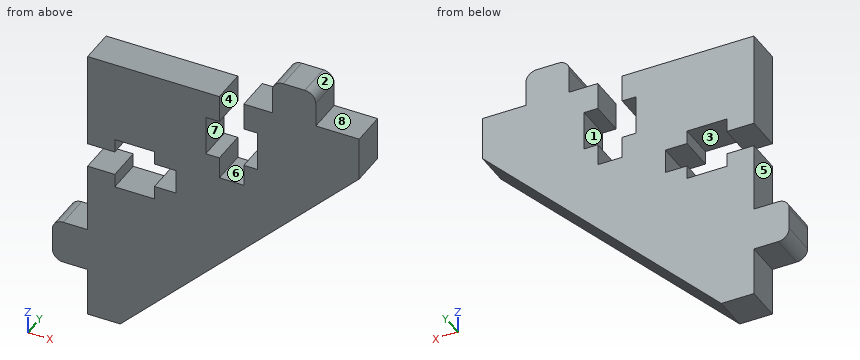
Autodesk Inventor part; units mm, degrees
ref_plane "YZ Plane" through (0, 0, 0) normal (1, 0, 0) x (0, 1, 0)
ref_plane "XZ Plane" through (0, 0, 0) normal (0, 1, 0) x (-1, 0, 0)
ref_plane "XY Plane" through (0, 0, 0) normal (0, 0, 1) x (1, 0, 0)
sketch "Sketch1" plane through (0, 0, 0) normal (0, 1, 0) x (-1, 0, 0)
  line L0 (0, -51.7) -> (0, 0)
  line L1 (0, 0) -> (-50, 0)
  line L2 (-50, 0) -> (-50, -8)
  line L3 (-50, -8) -> (-6, -51.7)
  line L4 (-6, -51.7) -> (0, -51.7)
  dimension "d0" = 51.7
  dimension "d1" = 50
  dimension "d2" = 8
  dimension "d3" = 6
extrude "Extrusion1" add sketch "Sketch1" along normal blind 6.5
sketch "Sketch2" plane through (0, 6.5, 0) normal (0, 1, 0) x (1, 0, 0)
  line L0 (0, 0) -> (50, 0)
  line L1 (50, 0) -> (50, 8)
  line L2 (34, 0) -> (42, 0)
  line L3 (42, 0) -> (42, -4.5)
  line L4 (40, -6.5) -> (36, -6.5)
  line L5 (34, -4.5) -> (34, 0)
  arc A0 (34, -4.5) -> (36, -6.5) centre (36, -4.5) ccw
  arc A1 (40, -6.5) -> (42, -4.5) centre (40, -4.5) ccw
  dimension "d6" = 2
  dimension "d7" = 8
  dimension "d8" = 6.5
  dimension "d9" = 8
extrude "Extrusion2" add sketch "Sketch2" against normal blind 6.5
sketch "Sketch3" plane through (0, 6.5, 0) normal (0, 1, 0) x (1, 0, 0)
  line L0 (0, 0) -> (34, 0)
  line L1 (34, 0) -> (34, -4.5)
  line L2 (24.25, 16.3) -> (28.75, 16.3)
  line L3 (28.75, 0) -> (24.25, 0)
  line L4 (31.25, 12.3) -> (31.25, 5)
  line L5 (21.75, 5) -> (21.75, 12.3)
  line L6 (21.75, 12.3) -> (24.25, 12.3)
  line L7 (28.75, 12.3) -> (31.25, 12.3)
  line L8 (24.25, 0) -> (24.25, 5)
  line L9 (24.25, 12.3) -> (24.25, 16.3)
  line L10 (31.25, 5) -> (28.75, 5)
  line L11 (24.25, 5) -> (21.75, 5)
  line L12 (28.75, 16.3) -> (28.75, 12.3)
  line L13 (28.75, 5) -> (28.75, 0)
  point P0 (26.5, 16.3)
  dimension "d12" = 4.5
  dimension "d13" = 5
  dimension "d14" = 7.3
  dimension "d15" = 4
  dimension "d16" = 2.5
  dimension "d17" = 7.5
extrude "Extrusion3" cut sketch "Sketch3" against normal through all
sketch "Sketch4" plane through (0, 6.5, 0) normal (0, 1, 0) x (1, 0, 0)
  line L0 (0, 51.7) -> (0, 0)
  line L1 (0, 0) -> (24.25, 0)
  line L2 (16.3, 22) -> (16.3, 17.5)
  line L3 (0, 17.5) -> (0, 22)
  line L4 (5, 24.5) -> (12.3, 24.5)
  line L5 (12.3, 15) -> (5, 15)
  line L6 (0, 22) -> (5, 22)
  line L7 (12.3, 22) -> (16.3, 22)
  line L8 (16.3, 17.5) -> (12.3, 17.5)
  line L9 (5, 17.5) -> (0, 17.5)
  line L10 (5, 15) -> (5, 17.5)
  line L11 (5, 22) -> (5, 24.5)
  line L12 (12.3, 24.5) -> (12.3, 22)
  line L13 (12.3, 17.5) -> (12.3, 15)
  point P0 (16.3, 19.75)
  dimension "d20" = 4.5
  dimension "d21" = 5
  dimension "d22" = 4
  dimension "d23" = 7.3
  dimension "d24" = 19.75
  dimension "d25" = 2.5
extrude "Extrusion4" cut sketch "Sketch4" against normal through all
sketch "Sketch5" plane through (0, 6.5, 0) normal (0, 1, 0) x (1, 0, 0)
  line L0 (16.3, 22) -> (16.3, 17.5)
  line L1 (0, 51.7) -> (0, 22)
  line L2 (0, 42.75) -> (-4.5, 42.75)
  line L3 (-6.5, 40.75) -> (-6.5, 36.75)
  line L4 (-4.5, 34.75) -> (0, 34.75)
  line L5 (0, 34.75) -> (0, 42.75)
  arc A0 (-4.5, 42.75) -> (-6.5, 40.75) centre (-4.5, 40.75) ccw
  arc A1 (-6.5, 36.75) -> (-4.5, 34.75) centre (-4.5, 36.75) ccw
  point P0 (16.3, 19.75)
  dimension "d28" = 2
  dimension "d29" = 8
  dimension "d30" = 6.5
  dimension "d31" = 15
extrude "Extrusion5" add sketch "Sketch5" against normal blind 6.5
properties part number "x_carryage_brace_top"
The listing builds one solid part. Answer for the finished solid, in the listing's coordinates (mm). Face numbers are marked on the shaded views. A direction names the side the tool comes from. Give positions to 0.01 mm unless a question says otherwise; leave off trailing zeros. Loops run counter-clockwise (first coordinate to the right, second up) from the corner with the lowest first, then second, coordinate; pieces in that order, holes last. Notation, with made-up numbers: (54, 61) - (107, 61) arc R25 ccw to (107, 98) - close; hole circle Ø1 at (-2, 87.5). An arc over 180 degrees is marked (long way). Answer as CSV lines item,"result". Start each with the question number.
Item 1: A cutting plane is placed at B-B on x = 9. Determine the outline of the cut face in (y, z).
Item 2: Find the intervals of material crossed by line 1 (X direction, y = 5.25, z = -4); line 2 (Z direction, x = 29.5, y = 4); line 3 (Z direction, x = 23.5, y = 4.25), in increasing order. Write a range as from..to.
Item 3: A cutting plane is placed at D-D on z = -45.5. Determine the outline of the cut face in (x, y).
Item 4: The mould has two halves that part along Z. Classify the marked faces 1, 2, 3 and 4: +Z half, -Z half, draft (parallel to the pull), parting line (faces both ways), or undercut.
Item 5: A cutting plane is placed at C-C on x = -1. Determine the outline of the cut face in (y, z), then the cut area to 3 significant figures.
Item 6: For the marked faces 5, 6, 7 and 8, determine the directions among +Z, -Z, +X, -X, +Y, -Y from which every point of the face is accessible in a straight line to the end or side of a thin tool.
Item 7: Each of these flat-tipped pins is pushed along its axis until it touches: pin 1 (2 mm diameter, centred on y = 4.5, z = -45.5, fed in from -X); pin 2 (2 mm diameter, centred on y = 2, z = -19, fed in from -X); pin 3 (2 mm diameter, centred on x = 47.5, y = 4.5, fed in from +Z). Where does it stop, or does it pass through?
Item 8: A cutting plane is placed at A-A on z = -3. Determine the outline of the cut face in (x, y).
Found:
1,outline,"(0, -48.72) - (6.5, -48.72) - (6.5, -24.5) - (0, -24.5) - close; (0, -15) - (6.5, -15) - (6.5, 0) - (0, 0) - close"
2,line 1,"x = 0..24.25, 28.75..50"
2,line 2,"z = -28.36..-12.3, -5..0"
2,line 3,"z = -34.32..-12.3, -5..0"
3,outline,"(0, 0) - (12.24, 0) - (12.24, 6.5) - (0, 6.5) - close"
4,face 1,"undercut"
4,face 2,"+Z half"
4,face 3,"undercut"
4,face 4,"draft"
5,outline,"(0, -42.75) - (6.5, -42.75) - (6.5, -34.75) - (0, -34.75) - close"
5,area,"52.0 mm^2"
6,face 5,"+Z, -X, +Y, -Y"
6,face 6,"+Z, +Y, -Y"
6,face 7,"+Y, -Y"
6,face 8,"+Z, +X, +Y, -Y"
7,pin 1,"stops at x = 0"
7,pin 2,"stops at x = 16.3"
7,pin 3,"stops at z = 0"
8,outline,"(0, 0) - (24.25, 0) - (24.25, 6.5) - (0, 6.5) - close; (28.75, 0) - (50, 0) - (50, 6.5) - (28.75, 6.5) - close"
